Check sheet for the modelled part. Datum: model origin and axes. Units: mm. A direction names the side the tool comes from. Round coordinates to 2 decimals unless told otherwise and drop trailing zeros. Loops run counter-clockwise (first coordinate to the right, second up) from the corner with the lowest first, then second, coordinate; pieces in that order, holes last. Notation, with made-up numbers: (86.25, -24) -> (124.25, -24) arc R8 cw to (124.25, -10) -> close; hole circle Ø3 at (3, 22.25). An arc over 180 degrees is marked (long way). One line per item, written item: value. Start each with the question number.
1. Set-up check for faces 1 (the face through (-19.1, -0.1, 0.4)), 2 (the face through (18, 2.825, 2)): record each of +Z, -Z, +X, -X, +Y, -Y from which the full face is reachable in a straight line by a thin tool's end or side.
2. Go/stop test with flat-tipped pins: pin 1 (3.5 mm diameter, centred on x = -17, z = 1, fed in from +Y) (3 decimals); pin 2 (1.5 mm diameter, centred on y = 1.5, z = 3.5, fed in from -X); pin 3 (3 mm diameter, centred on x = 7, z = -0.5, fed in from -Y). Record where each tip stops, or that it passes through.
3. Material ranges on L1, parallel to X at y = 1.95, z = 0; L2, parallel to X at y = 3.75, z = -3.25; L3, parallel to Z at x = 16, y = 3.5, recorded low to high.
4. Cross-section at C-C on z = 0.5. Count the separate pieces of the cut face and the enclosed holes in it, then the cut area to 3 significant figures.
5. Cross-section at A-A on y = 3.25. Record the cut outline in (x, z) (3 decimals).
6. Cross-section at B-B on x = 10.5. Record the cut outline in (y, z), then the cut area to 3 significant figures.
7. Release check for a two-part mould opening along X. For faces 3 (the face through (19.1, -0.1, 0.4)), 4 (the face through (0, 6, 0)), 5 (the face through (-21.914, 3.597, -0.133)), 6 (the face through (12.83, 3.999, 1.726)) record: +X half, -X half, draft (parallel to the pull), parting line (faces both ways), or undercut.
from build123d import *

# Parameters (mm, degrees)
BOSS_EXTRUDE1_DEPTH = 4.5
BOSS_EXTRUDE2_DEPTH = 1.5
CUT_EXTRUDE1_DEPTH  = 1.2375
SKETCH6_R           = 2.125
BOSS_EXTRUDE3_DEPTH = 1.5875
BOSS_EXTRUDE4_START = 1.778
SKETCH7_R           = 3.25
SKETCH7_R_2         = 2.125
BOSS_EXTRUDE4_DEPTH = 1.778
FILLET2_R           = 0.79375
FILLET3_R           = 0.79375


with BuildPart() as part:
    # Sketch1 → Boss-Extrude1 (new body)
    with BuildSketch(Plane(origin=(0, 0, 0), x_dir=(1, 0, 0), z_dir=(0, 1, 0))):
        with BuildLine():
            Line((-15.875, 6.04), (15.875, 6.04))
            ThreePointArc((15.875, 6.04), (21.915, 0), (15.875, -6.04))
            Line((15.875, -6.04), (-15.875, -6.04))
            ThreePointArc((-15.875, -6.04), (-21.915, 0), (-15.875, 6.04))
        make_face()
        Polygon((-13.854274058, 3.5), (-17.895725942, 3.5), (-19.916451884, 0), (-17.895725942, -3.5), (-13.854274058, -3.5), (-11.833548116, 0), align=None, mode=Mode.SUBTRACT)
        Polygon((17.895725942, 3.5), (13.854274058, 3.5), (11.833548116, 0), (13.854274058, -3.5), (17.895725942, -3.5), (19.916451884, 0), align=None, mode=Mode.SUBTRACT)
    extrude(amount=BOSS_EXTRUDE1_DEPTH)

    # Sketch2 → Boss-Extrude2 (add)
    with BuildSketch(Plane(origin=(0, 4.5, 0), x_dir=(1, 0, 0), z_dir=(0, 1, 0))):
        with BuildLine():
            Line((15.875, 6.04), (-15.875, 6.04))
            ThreePointArc((-15.875, 6.04), (-21.915, 0), (-15.875, -6.04))
            Line((-15.875, -6.04), (15.875, -6.04))
            ThreePointArc((15.875, -6.04), (21.915, 0), (15.875, 6.04))
        make_face()
        Polygon((19.916451884, 0), (17.895725942, 3.5), (13.854274058, 3.5), (11.833548116, 0), (13.854274058, -3.5), (17.895725942, -3.5), align=None, mode=Mode.SUBTRACT)
        Polygon((-17.895725942, 3.5), (-19.916451884, 0), (-17.895725942, -3.5), (-13.854274058, -3.5), (-11.833548116, 0), (-13.854274058, 3.5), align=None, mode=Mode.SUBTRACT)
    extrude(amount=BOSS_EXTRUDE2_DEPTH)

    # Sketch3 → Cut-Extrude1 (cut)
    with BuildSketch(Plane.XZ):
        with BuildLine():
            Line((15.875, 6.04), (-15.875, 6.04))
            ThreePointArc((-15.875, 6.04), (-21.915, 0), (-15.875, -6.04))
            Line((-15.875, -6.04), (15.875, -6.04))
            ThreePointArc((15.875, -6.04), (21.915, 0), (15.875, 6.04))
        make_face()
    extrude(amount=-CUT_EXTRUDE1_DEPTH, mode=Mode.SUBTRACT)

    # Sketch6 → Boss-Extrude3 (add)
    with BuildSketch(Plane.XZ.offset(-1.2375)):
        Polygon((13.854274058, 3.5), (11.833548116, 0), (13.854274058, -3.5), (17.895725942, -3.5), (19.916451884, 0), (17.895725942, 3.5), align=None)
        with Locations(Location((15.875, 0, 0), (0, 0, 270))):
            Circle(SKETCH6_R, mode=Mode.SUBTRACT)
    boss_extrude3 = extrude(amount=-BOSS_EXTRUDE3_DEPTH)

    # Sketch7 → Boss-Extrude4 (add)
    with BuildSketch(Plane.XZ.offset(-1.2375).offset(BOSS_EXTRUDE4_START)):
        with Locations(Location((15.875, 0, 0), (0, 0, 270))):
            Circle(SKETCH7_R)
        with Locations(Location((15.875, 0, 0), (0, 0, 270))):
            Circle(SKETCH7_R_2, mode=Mode.SUBTRACT)
    boss_extrude4 = extrude(amount=-BOSS_EXTRUDE4_DEPTH)

    # Mirror1: Boss-Extrude3, Boss-Extrude4 across plane
    add(boss_extrude3.mirror(Plane(origin=(0, 0, 0), x_dir=(0, 0, 1), z_dir=(1, 0, 0))))
    add(boss_extrude4.mirror(Plane(origin=(0, 0, 0), x_dir=(0, 0, 1), z_dir=(1, 0, 0))))

    # Fillet2
    fillet2_edges = [part.edges().sort_by_distance(p)[0] for p in [
        (21.915, 1.2375, 0),
        (0, 1.2375, -6.04),
        (-21.915, 1.2375, 0),
        (0, 1.2375, 6.04),
        (15.875, 1.2375, 3.25),
        (-15.875, 1.2375, 3.25),
    ]]
    fillet(fillet2_edges, radius=FILLET2_R)

    # Fillet3
    fillet3_edges = [part.edges().sort_by_distance(p)[0] for p in [
        (21.915, 6, 0),
        (0, 6, -6.04),
        (-21.915, 6, 0),
        (0, 6, 6.04),
        (18.906088913, 6, 1.75),
        (15.875, 6, 3.5),
        (12.843911087, 6, 1.75),
        (12.843911087, 6, -1.75),
        (15.875, 6, -3.5),
        (18.906088913, 6, -1.75),
        (-15.875, 6, -3.5),
        (-12.843911087, 6, -1.75),
        (-12.843911087, 6, 1.75),
        (-15.875, 6, 3.5),
        (-18.906088913, 6, 1.75),
        (-18.906088913, 6, -1.75),
    ]]
    fillet(fillet3_edges, radius=FILLET3_R)


solid = part.part
Taken from the geometry:
1. face 1: -Y
1. face 2: +Y
2. pin 1: stops at y = 2.825
2. pin 2: stops at x = -21.18
2. pin 3: stops at y = 1.24
3. L1: x = -21.91 to -18, -13.75 to 13.75, 18 to 21.91
3. L2: x = -20.97 to -18.04, -13.71 to 13.71, 18.04 to 20.97
3. L3: z = -6.04 to -3.5, 3.5 to 6.04
4. separate pieces: 3
4. enclosed holes: 0
4. area: 155 mm2
5. outline: (-15.875, -6.04) -> (15.875, -6.04) arc R6.04 ccw to (15.875, 6.04) -> (-15.875, 6.04) arc R6.04 ccw to start; hole (-19.916, 0) -> (-17.896, -3.5) -> (-13.854, -3.5) -> (-11.834, 0) -> (-13.854, 3.5) -> (-17.896, 3.5) -> close; hole (11.834, 0) -> (13.854, -3.5) -> (17.896, -3.5) -> (19.916, 0) -> (17.896, 3.5) -> (13.854, 3.5) -> close
6. outline: (1.24, -5.25) arc R0.79 ccw to (2.03, -6.04) -> (5.21, -6.04) arc R0.79 ccw to (6, -5.25) -> (6, 5.25) arc R0.79 ccw to (5.21, 6.04) -> (2.03, 6.04) arc R0.79 ccw to (1.24, 5.25) -> close
6. area: 57.0 mm2
7. face 3: undercut
7. face 4: draft
7. face 5: -X half
7. face 6: undercut
